Geometry: final body of the model. Coordinates: model frame, mm. A direction names the side the tool comes from. Give positions to 0.01 mm unless a question says otherwise; leave off trailing zeros. Write each loop counter-clockwise with the first axis right and the second up, starting at its lowest first coordinate (ties: lowest second). Pieces come first, ordered by that corner, then holes. Notation, with made-up numbers: (12.25, -37.5) -> (59.25, -37.5) arc R12 cw to (59.25, -27.5) -> close; hole circle Ø1 at (23, 33). An arc over 180 degrees is marked (long way). Answer as a JSON object with one key per item and string values. Group by question number.
(1) Set-up query: faces 1 (the face through (-45, -12, -30)), 2 (the face through (-43, -6, -29.7)), 3 (the face through (0, 2, 0)), 4 (the face through (-19, -10, 11.3)). Return all of +Z, -Z, +X, -X, +Y, -Y with unobstructed straight access to the full face (end or side cutting, diameter ignored); none if empty.
(2) Material intervals for probe 1 along Z at (x, y) = (0, 4.7); probe 2 along Z at (x, y) = (-19.2, -15); probe 3 along Y at (x, z) = (-18.6, -34), sorted ascending.
(3) Section query B-B on z = 30. Output: boundary loops of the cut face in (x, y), plus the area to 3 significant figures.
(4) Section query A-A on y = -10. Output: boundary loops of the cut face in (x, z), plus the area to 3 significant figures.
(5) Section query C-C on x = -27.5. Output: boundary loops of the cut face in (y, z), plus the area to 3 significant figures.
(6) Section query D-D on x = -49.5. Output: boundary loops of the cut face in (y, z), plus the area to 3 significant figures.
(7) Draft query along X for faces 5 (the face through (-20.5, -10, -34)), 6 (the face through (-19, -14.1, -32.8)), 7 (the face through (-47.5, -6, -30)). Return one class per face: +X half, -X half, draft (parallel to the pull), parting line (faces both ways), or undercut.
(8) Contact query for flat-ended pins moving along their axis: pin 1 Ø4 at (x, z) = (-49.5, 6.5) entering from +Y; pin 2 Ø3 at (y, z) = (-7, 11) entering from +X; pin 3 Ø0.9 at (x, y) = (-19, -5.5) entering from +Z; pin 4 Ø1.8 at (y, z) = (-5, 15.6) entering from +X. Output: stop coordinate, or through.
Autodesk Inventor part; units mm, degrees
ref_plane "Work Plane1" through (-17.5, 0, -9.2) normal (1, 0, 0) x (0, 0, -1)
ref_plane "Work Plane2" through (16, 0, 0) normal (1, 0, 0) x (0, 1, 0)
ref_plane "XZ Plane" through (0, 0, 0) normal (0, 1, 0) x (-1, 0, 0)
sketch "Sketch1" plane through (0, 0, 0) normal (0, 1, 0) x (-1, 0, 0)
  circle A0 centre (0, 0) radius 63.5
  circle A1 centre (0, -7.2) radius 0.6
  circle A2 centre (3.5, -7.2) radius 0.6
  circle A3 centre (-3.5, -7.2) radius 0.6
  circle A4 centre (7.2, 3.5) radius 0.6
  circle A5 centre (7.2, 0) radius 0.6
  circle A6 centre (7.2, -3.5) radius 0.6
  circle A7 centre (-3.5, 7.2) radius 0.6
  circle A8 centre (0, 7.2) radius 0.6
  circle A9 centre (3.5, 7.2) radius 0.6
  circle A10 centre (-7.2, -3.5) radius 0.6
  circle A11 centre (-7.2, 0) radius 0.6
  circle A12 centre (-7.2, 3.5) radius 0.6
  circle A13 centre (0, 0) radius 10.4
  circle A14 centre (0, 0) radius 12
  circle A15 centre (0, 0) radius 4
  dimension "d0" = 127
  dimension "d1" = 7.2
  dimension "d2" = 1.2
  dimension "d3" = 3.5
  dimension "d4" = 3.5
  dimension "d5" = 1.2
  dimension "d6" = 1.2
  dimension "d9" = 360
  dimension "d15" = 20.8
  dimension "d16" = 24
  dimension "d19" = 8
extrude "Extrusion1" add sketch "Sketch1" along normal blind 3 contours A0 | A13 | A14
extrude "Extrusion2" add sketch "Sketch1" along normal blind 6 contours A1 | A2 | A3 | A4 | A5 | A6 | A7 | A8 | A9 | A10 | A11 | A12
extrude "Extrusion3" add sketch "Sketch1" along normal blind 6 contours A14
extrude "Extrusion4" add sketch "Sketch1" along normal blind 2 contours A15
sketch "Sketch2" plane through (0, 0, 0) normal (0, -1, 0) x (1, 0, 0)
  line L0 (-17.5, 11.3) -> (-44.5, 11.3) construction
  line L1 (-44.5, 11.3) -> (-44.5, -29.7) construction
  line L2 (-44.5, -29.7) -> (-17.5, -29.7) construction
  line L3 (-17.5, -29.7) -> (-17.5, 11.3) construction
  line L4 (-47.5, 14.3) -> (-47.5, 8.3)
  line L5 (-47.5, 8.3) -> (-44.5, 8.3)
  line L6 (-44.5, 8.3) -> (-44.5, 11.3)
  line L7 (-17.5, 11.3) -> (-17.5, 19.3)
  line L8 (-17.5, 19.3) -> (-20.5, 19.3)
  line L9 (-20.5, 19.3) -> (-20.5, 11.3)
  line L10 (-20.5, 11.3) -> (-17.5, 11.3)
  line L11 (-44.5, -9.2) -> (-17.5, -9.2) construction
  line L12 (-17.5, -29.7) -> (-44.5, -29.7) construction
  line L13 (-44.5, -29.7) -> (-41.5, -29.7)
  line L14 (-41.5, -29.7) -> (-41.5, -32.7)
  line L15 (-41.5, -32.7) -> (-47.5, -32.7)
  line L16 (-47.5, -32.7) -> (-47.5, -26.7)
  line L17 (-47.5, -26.7) -> (-44.5, -26.7)
  line L18 (-44.5, -26.7) -> (-44.5, -29.7)
  line L19 (-17.5, -29.7) -> (-17.5, -37.7)
  line L20 (-17.5, -37.7) -> (-20.5, -37.7)
  line L21 (-20.5, -37.7) -> (-20.5, -29.7)
  line L22 (-20.5, -29.7) -> (-17.5, -29.7)
  line L23 (-47.5, 14.3) -> (-44.5, 14.3)
  line L24 (-44.5, 14.3) -> (-44.5, 11.3)
  point P0 (0, 0)
  point P1 (-41.5, 11.3)
  point P2 (-31, 0)
  dimension "d22" = 27
  dimension "d23" = 41
  dimension "d24" = 3
  dimension "d28" = 6
  dimension "d29" = 3
  dimension "d31" = 8
  dimension "d32" = 3
  dimension "d33" = 8
  dimension "d34" = 90
  dimension "d50" = 44.5
  dimension "d51" = 29.7
  dimension "d52" = 3
  dimension "d53" = 3
extrude "Extrusion5" add sketch "Sketch2" along normal blind 12 contours L23 L24 L6 L5 L4 | L13 L14 L15 L16 L17 L18
extrude "Extrusion6" add sketch "Sketch2" along normal blind 20 contours L10 L9 L8 L7 | L19 L20 L21 L22
ref_plane "Work Plane1" through (-17.5, 0, -9.2) normal (1, 0, 0) x (0, 0, -1)
sketch "Sketch3" plane through (-17.5, 0, -9.2) normal (1, 0, 0) x (0, 0, -1)
  line L0 (0, 0) -> (0, -20) construction
  line L1 (0, 0) -> (20, 0) construction
  line L2 (28.5, -20) -> (20.5, -20)
  line L3 (24.8, -20) -> (24.8, 0) construction
  line L4 (24.8, -10) -> (0, -10) construction
  point P0 (-9.2, 0)
  point P1 (0, 0)
  point P2 (24.8, -15)
  point P3 (24.8, -5)
  point P4 (-24.8, -15)
  point P5 (-24.8, -5)
  dimension "d39" = 20
  dimension "d40" = 90
  dimension "d41" = 24.8
  dimension "d42" = 10
hole "Hole1" at (-17.5, -15, 15.6) at (-17.5, -5, 15.6) at (-17.5, -5, -34) at (-17.5, -15, -34) direction (-1, 0, 0) diameter 3 depth 3
sketch "Sketch4" plane through (0, 0, 0) normal (0, -1, 0) x (1, 0, 0)
  point P0 (0, 0)
  point P1 (44.45, 0)
  point P2 (31.4309, 31.4309)
  point P3 (0, 44.45)
  point P4 (-31.4309, 31.4309)
  point P5 (-44.45, 0)
  point P6 (-31.4309, -31.4309)
  point P7 (0, -44.45)
  point P8 (31.4309, -31.4309)
  dimension "d56" = 360
hole "Hole2" at (-31.4309, 0, 31.4309) at (0, 0, 44.45) at (31.4309, 0, 31.4309) at (44.45, 0, 0) at (31.4309, 0, -31.4309) at (0, 0, -44.45) direction (0, 1, 0) diameter 12 end through all
ref_plane "Work Plane2" through (16, 0, 0) normal (1, 0, 0) x (0, 1, 0)
split "Split1" plane through (16, 0, 0) removes the side toward (1, 0, 0)
properties part number "pan_platform"
Answer list:
{
 "1": {"face 1": "+Z, -Z, -X, -Y", "face 2": "+Z, +X, -Y", "face 3": "+Y", "face 4": "+X, -Y"},
 "2": {"probe 1": "-12 to -10.4, -7.8 to -6.6, 6.6 to 7.8, 10.4 to 12", "probe 2": "-37.7 to -35.5, -32.5 to -29.7, 11.3 to 14.1, 17.1 to 19.3", "probe 3": "-20 to -16.5, -13.5 to -6.5, -3.5 to 3"},
 "3": {"outline": "(-55.97, 0) -> (-37.26, 0) -> (-37.26, 3) -> (-55.97, 3) -> close; (-25.6, 0) -> (16, 0) -> (16, 3) -> (-25.6, 3) -> close", "area": "181 mm2"},
 "4": {"outline": "(-47.5, -32.7) -> (-41.5, -32.7) -> (-41.5, -29.7) -> (-44.5, -29.7) -> (-44.5, -26.7) -> (-47.5, -26.7) -> close; (-47.5, 8.3) -> (-44.5, 8.3) -> (-44.5, 14.3) -> (-47.5, 14.3) -> close; (-20.5, -37.7) -> (-17.5, -37.7) -> (-17.5, -29.7) -> (-20.5, -29.7) -> close; (-20.5, 11.3) -> (-17.5, 11.3) -> (-17.5, 19.3) -> (-20.5, 19.3) -> close", "area": "93.0 mm2"},
 "5": {"outline": "(0, -57.24) -> (3, -57.24) -> (3, 26.9) -> (0, 26.9) -> close; (0, 35.96) -> (3, 35.96) -> (3, 57.24) -> (0, 57.24) -> close", "area": "316 mm2"},
 "6": {"outline": "(0, -39.77) -> (3, -39.77) -> (3, 39.77) -> (0, 39.77) -> close", "area": "239 mm2"},
 "7": {"face 5": "undercut", "face 6": "draft", "face 7": "-X half"},
 "8": {"pin 1": "y = 3", "pin 2": "x = -17.5", "pin 3": "z = 19.3", "pin 4": "through"}
}
